```python
from build123d import *

# Parameters (mm, degrees)
SKETCH120_W     = 40
SKETCH120_H     = 40
SKETCH120_R     = 1.7
SKETCH120_R_2   = 2.1
PAD062_DEPTH    = 6
CHAMFER017_SIZE = 3
POCKET021_DEPTH = 4
SKETCH122_W     = 44.906031
SKETCH122_H     = 45.853912
POCKET022_DEPTH = 2
CHAMFER018_SIZE = 0.4
SKETCH123_W     = 14
SKETCH123_H     = 10
POCKET023_DEPTH = 6.001
CHAMFER019_SIZE = 1


with BuildPart() as part:
    # Sketch120 → Pad062 (new body)
    with BuildSketch(Plane.XZ):
        with Locations((0, 20)):
            Rectangle(SKETCH120_W, SKETCH120_H)
        with Locations((-8.5, 34)):
            Circle(SKETCH120_R, mode=Mode.SUBTRACT)
        with Locations((0, 30)):
            Circle(SKETCH120_R_2, mode=Mode.SUBTRACT)
        with Locations((0, 17)):
            Circle(SKETCH120_R_2, mode=Mode.SUBTRACT)
    extrude(amount=PAD062_DEPTH)

    # Chamfer017
    chamfer017_edges = [part.edges().sort_by_distance(p)[0] for p in [
        (-20, -3, 40),
        (20, -3, 40),
        (20, -3, 0),
        (-20, -3, 0),
    ]]
    chamfer(chamfer017_edges, length=CHAMFER017_SIZE)

    # Sketch121 (on Face5 of Chamfer017) → Pocket021 (cut)
    with BuildSketch(Plane.XZ.offset(6)):
        with BuildLine():
            ThreePointArc((-12.7, 34), (-8.5, 29.8), (-4.3, 34))
            Line((-4.3, 34), (-4.3, 40))
            ThreePointArc((-4.3, 40), (-8.5, 44.2), (-12.7, 40))
            Line((-12.7, 40), (-12.7, 34))
        make_face()
    extrude(amount=-POCKET021_DEPTH, mode=Mode.SUBTRACT)

    # Sketch122 (on Face5 of Pocket021) → Pocket022 (cut)
    with BuildSketch(Plane.XZ.offset(6)):
        with Locations((-0.23733, 20.575699)):
            Rectangle(SKETCH122_W, SKETCH122_H)
        with BuildLine():
            ThreePointArc((4.2, 30), (0, 34.2), (-4.2, 30))
            Line((-4.2, 30), (-4.2, 17))
            ThreePointArc((-4.2, 17), (0, 12.8), (4.2, 17))
            Line((4.2, 17), (4.2, 30))
        make_face(mode=Mode.SUBTRACT)
    extrude(amount=-POCKET022_DEPTH, mode=Mode.SUBTRACT)

    # Chamfer018
    chamfer018_edges = [part.edges().sort_by_distance(p)[0] for p in [
        (-10.2, -2, 34),
        (-2.1, -6, 30),
        (-2.1, -6, 17),
        (-2.1, 0, 17),
        (-2.1, 0, 30),
        (-10.2, 0, 34),
        (0, -6, 34.2),
        (0, -4, 34.2),
        (-4.3, -3, 40),
        (-12.7, -3, 40),
    ]]
    chamfer(chamfer018_edges, length=CHAMFER018_SIZE)

    # Sketch123 → Pocket023 (cut, through all)
    with BuildSketch(Plane.XZ):
        with Locations((0, 5)):
            Rectangle(SKETCH123_W, SKETCH123_H)
    extrude(amount=POCKET023_DEPTH, mode=Mode.SUBTRACT)

    # Chamfer019
    chamfer019_edges = [part.edges().sort_by_distance(p)[0] for p in [
        (7, -2, 10),
        (-7, -2, 10),
        (7, -2, 0),
        (-7, -2, 0),
    ]]
    chamfer(chamfer019_edges, length=CHAMFER019_SIZE)


with BuildPart() as part_1:
    # Body053 placement: moved
    add(part.part.moved(Location((0, -3, 192))))


solid = part_1.part
```
Verification items for the finished model (mm, model axes). A direction names the side the tool comes from. Round coordinates to 2 decimals unless told otherwise and drop trailing zeros. Order: outer loops, then holes, each group sorted by start corner. A loop starts at its lowest first (then second) coordinate and runs counter-clockwise, first axis right, second up. Notation, with made-up numbers: (64.25, 41) - (82.25, 41) arc R20 ccw to (82.25, 55) - close; hole circle Ø2 at (52.25, -28.5). An arc over 180 degrees is marked (long way). Use CSV: the item, a comma, the result in double quotes.
(1) Section check B-B on x = -8.5. Record the boundary of the cut face in (y, z).
Entries:
outline,"(-7, 192) - (-3, 192) - (-3, 223.9) - (-3.4, 224.3) - (-4.6, 224.3) - (-5, 223.9) - (-5, 221.8) - (-7, 221.8) - close; (-5, 228.1) - (-4.6, 227.7) - (-3.4, 227.7) - (-3, 228.1) - (-3, 232) - (-5, 232) - close"
(2) Access from +Z, -Z, +X, -X, +Y, -Y to the whole of each face (thin tool, end or side, straight path). Record for faces 4 (the face through (-4.3, -6, 229)), 5 (the face through (-0.1, -8, 204.8)), 6 (the face through (19, -5, 194)), 7 (the face through (7, -5, 197)).
Entries:
face 4,"+Z, -Y"
face 5,"-Z, -Y"
face 6,"-Z, +X, +Y, -Y"
face 7,"-Z, +Y, -Y"
(3) Section check C-C on x = 0. Record the boundary of the cut face in (y, z).
Entries:
outline,"(-9, 205.2) - (-8.6, 204.8) - (-7.4, 204.8) - (-7, 204.4) - (-7, 202) - (-3, 202) - (-3, 206.5) - (-3.4, 206.9) - (-8.6, 206.9) - (-9, 206.5) - close; (-9, 211.5) - (-8.6, 211.1) - (-3.4, 211.1) - (-3, 211.5) - (-3, 219.5) - (-3.4, 219.9) - (-8.6, 219.9) - (-9, 219.5) - close; (-9, 224.5) - (-8.6, 224.1) - (-3.4, 224.1) - (-3, 224.5) - (-3, 232) - (-7, 232) - (-7, 226.6) - (-7.4, 226.2) - (-8.6, 226.2) - (-9, 225.8) - close"
(4) Thickness scan on probe 1 along Z at (x, y) = (0, -6.75); probe 2 along X at (y, z) = (-4.3, 226); probe 3 along Z at (x, y) = (-8.5, -3.7). Record the ranges inside material, lowest first. Write a range as from..to.
Entries:
probe 1,"202..206.9, 211.1..219.9, 224.1..232"
probe 2,"-20..-10.2, -6.8..20"
probe 3,"192..224.3, 227.7..232"
(5) Section check A-A on y = -4. Record the boundary of the cut face in (x, z).
Entries:
outline,"(-20, 195) - (-17, 192) - (-8, 192) - (-7, 193) - (-7, 201) - (-6, 202) - (6, 202) - (7, 201) - (7, 193) - (8, 192) - (17, 192) - (20, 195) - (20, 229) - (17, 232) - (-17, 232) - (-20, 229) - close; hole circle Ø3.4 at (-8.5, 226); hole circle Ø4.2 at (0, 209); hole circle Ø4.2 at (0, 222)"
(6) Gauge pin test, flat ends, axial feed: pin 1 Ø3 at (x, y) = (-3, -5.5) entering from -Z; pin 2 Ø0.6 at (y, z) = (-8, 218.5) entering from -X; pin 3 Ø4.5 at (x, z) = (-8, 227.5) entering from -Y; pin 4 Ø3 at (x, z) = (-8.5, 226) entering from +Y. Record the tip position at first contact, or that the pin passes through.
Entries:
pin 1,"z = 202"
pin 2,"x = -4.2"
pin 3,"y = -5"
pin 4,"through"
(7) Mould release check, pull along Z, two halves, no side actions. Record for faces 1 (the face through (-18, -5, 193)), 2 (the face through (-4.2, -8, 216)), 3 (the face through (-0.273, -5.964, 224.082)): released by +Z, released by -Z, zero draft, split by the parting line, or undercut.
Entries:
face 1,"released by -Z"
face 2,"zero draft"
face 3,"undercut"
(8) Section check D-D on z = 212. Record the boundary of the cut face in (x, y), and give its area (3 significant figures).
Entries:
outline,"(-20, -7) - (-4.6, -7) - (-4.2, -7.4) - (-4.2, -8.6) - (-3.8, -9) - (3.8, -9) - (4.2, -8.6) - (4.2, -7.4) - (4.6, -7) - (20, -7) - (20, -3) - (-20, -3) - close"
area,"177 mm^2"
